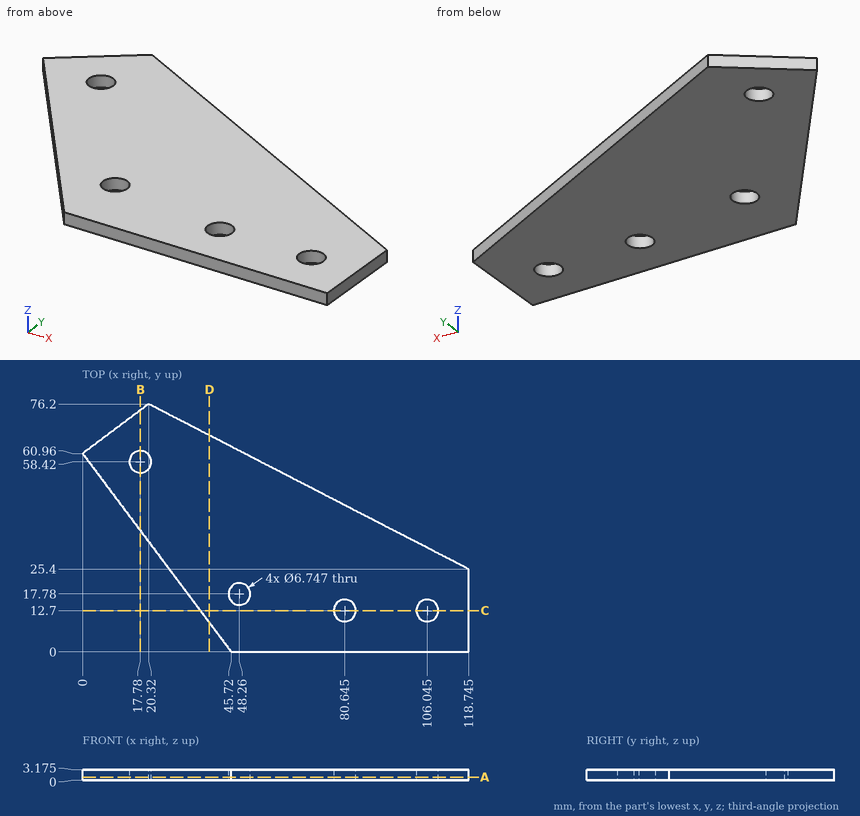
Check sheet for the drawn part. Datum: minimum x, y, z corner. Units: mm. Round coordinates to 2 decimals unless told otherwise and drop trailing zeros. Write each loop counter-clockwise with the first axis right and the second up, starting at its lowest first coordinate (ties: lowest second). Pieces come first, ordered by that corner, then holes. Notation, with made-up numbers: (-17, -29) -> (-11, -29) arc R14 ccw to (-11, -20) -> close; hole circle Ø8 at (62, 50). An arc over 180 degrees is marked (long way). Write each question's results on one line, items separated by ' | '.
Q1. Sectioned sample at B-B, the plane x = 17.78. Record the boundary of the cut face in (y, z) (1 decimal).
Derived:
outline: (37.3, 0) -> (55, 0) -> (55, 3.2) -> (37.3, 3.2) -> close; (61.8, 0) -> (74.3, 0) -> (74.3, 3.2) -> (61.8, 3.2) -> close
Q2. Sectioned sample at C-C, the plane y = 12.7. Record the boundary of the cut face in (x, z) (1 decimal).
Derived:
outline: (36.2, 0) -> (77.3, 0) -> (77.3, 3.2) -> (36.2, 3.2) -> close; (84, 0) -> (102.7, 0) -> (102.7, 3.2) -> (84, 3.2) -> close; (109.4, 0) -> (118.7, 0) -> (118.7, 3.2) -> (109.4, 3.2) -> close
Q3. Go/stop test with flat-tipped pins: pin 1 Ø8 at (x, y) = (80.65, 12.7) entering from +Z (3 decimals); pin 2 Ø1 at (x, z) = (37, 1.5) entering from +Y; pin 3 Ø5.5 at (x, y) = (17.78, 58.42) entering from +Z; pin 4 Ø1 at (y, z) = (36, 2.5) entering from -X (1 decimal). Record where each tip stops, or that it passes through.
Derived:
pin 1: stops at z = 3.175 | pin 2: stops at y = 67.85 | pin 3: passes through | pin 4: stops at x = 18.3
Q4. Sectioned sample at D-D, the plane x = 39. Record the boundary of the cut face in (y, z) (1 decimal), and give its area (3 significant figures).
Derived:
outline: (9, 0) -> (66.6, 0) -> (66.6, 3.2) -> (9, 3.2) -> close | area: 183 mm²
Q5. Thickness scan on probe 1 along X at (y, z) = (11, 0.4) (1 decimal); probe 2 along Y at (x, z) = (107, 0.6) (1 decimal); probe 3 along Y at (x, z) = (17.78, 1) (1 decimal). Record the ranges inside material, lowest first.
Derived:
probe 1: x = 37.5 to 77.7, 83.6 to 103.1, 109 to 118.7 | probe 2: y = 0 to 9.5, 15.9 to 31.5 | probe 3: y = 37.3 to 55, 61.8 to 74.3
Q6. Sectioned sample at A-A, the plane z = 0.9. Record the boundary of the cut face in (x, y) (1 decimal).
Derived:
outline: (0, 61) -> (45.7, 0) -> (118.7, 0) -> (118.7, 25.4) -> (20.3, 76.2) -> close; hole circle Ø6.7 at (17.8, 58.4); hole circle Ø6.7 at (48.3, 17.8); hole circle Ø6.7 at (80.6, 12.7); hole circle Ø6.7 at (106, 12.7)
